Verification items for the finished model (mm, model axes). A direction names the side the tool comes from. Give positions to 0.01 mm unless a question says otherwise; leave off trailing zeros. Write each loop counter-clockwise with the first axis right and the second up, starting at its lowest first coordinate (ties: lowest second). Pieces come first, ordered by that corner, then holes. Notation, with made-up numbers: (13, 22.25) - (20, 22.25) arc R24 cw to (20, 56.25) - close; hole circle Ø10 at (-19.5, 53.5). An arc over 180 degrees is marked (long way). Put each result on its own line as item: value.
from build123d import *

# Parameters (mm, degrees)
IZIM1_R                     = 35
Y_KSEKLIK_EKSTR_ZYON1_DEPTH = 10
IZIM2_W                     = 12
IZIM2_H                     = 12
KES_EKSTR_ZYON1_DEPTH       = 16
RADYUS1_R                   = 3


with BuildPart() as part:
    # Çizim1 → Yükseklik-Ekstrüzyon1 (new body)
    with BuildSketch(Plane.XY):
        Circle(IZIM1_R)
    extrude(amount=Y_KSEKLIK_EKSTR_ZYON1_DEPTH)

    # Çizim2 → Kes-Ekstrüzyon1 (cut)
    with BuildSketch(Plane(origin=(0, 0, 0), x_dir=(-1, 0, 0), z_dir=(0, 0, -1))):
        with Locations((0, 29)):
            Rectangle(IZIM2_W, IZIM2_H)
        with Locations((0, -29)):
            Rectangle(IZIM2_W, IZIM2_H)
    extrude(amount=-KES_EKSTR_ZYON1_DEPTH, mode=Mode.SUBTRACT)

    # Radyus1
    radyus1_edges = [part.edges().sort_by_distance(p)[0] for p in [
        (-6, 34.481879299, 5),
        (6, 34.481879299, 5),
        (6, 23, 5),
        (-6, 23, 5),
        (-6, -34.481879299, 5),
        (-6, -23, 5),
        (6, -34.481879299, 5),
        (6, -23, 5),
    ]]
    fillet(radyus1_edges, radius=RADYUS1_R)


solid = part.part
Q1. Section check C-C, the plane x = -11.5. Record the cut outline in (y, z).
Answers follow:
outline: (-33.06, 0) - (33.06, 0) - (33.06, 10) - (-33.06, 10) - close
Q2. Go/stop test with flat-tipped pins: pin 1 Ø4 at (y, z) = (29, 3) entering from +X; pin 2 Ø5 at (y, z) = (27.5, 3.5) entering from -X; pin 3 Ø4 at (y, z) = (-27.5, 3.5) entering from +X. Record where each tip stops, or that it passes through.
Answers follow:
pin 1: stops at x = 22.27
pin 2: stops at x = -24.49
pin 3: stops at x = 23.97
Q3. Set-up check for faces 4 (the face through (-5.14, -23.9, 5.07)), 5 (the face through (0, 0, 10)), 6 (the face through (-6, 28, 5)): record each of +Z, -Z, +X, -X, +Y, -Y from which the full face is reachable in a straight line by a thin tool's end or side.
Answers follow:
face 4: +Z, -Z, -Y
face 5: +Z, +X, -X, +Y, -Y
face 6: +Z, -Z, +Y
Q4. Section check A-A, the plane z = 7. Record the cut outline in (x, y), plus the area to 3 significant figures.
Answers follow:
outline: (-9.84, -33.59) arc R3 ccw to (-6, -30.71) - (-6, -26) arc R3 cw to (-3, -23) - (3, -23) arc R3 cw to (6, -26) - (6, -30.71) arc R3 ccw to (9.84, -33.59) arc R35 ccw to (9.84, 33.59) arc R3 ccw to (6, 30.71) - (6, 26) arc R3 cw to (3, 23) - (-3, 23) arc R3 cw to (-6, 26) - (-6, 30.71) arc R3 ccw to (-9.84, 33.59) arc R35 ccw to start
area: 3,560 mm2
Q5. Scan lines: line 1 along X through (y, z) = (27, 4); line 2 along X through (y, z) = (-26, 9.75); line 3 along Y through (x, z) = (-26.5, 6.25). Record each from-to range of solid material in increasing order.
Answers follow:
line 1: x = -22.27 to -6, 6 to 22.27
line 2: x = -23.43 to -6, 6 to 23.43
line 3: y = -22.86 to 22.86
Q6. Section check B-B, the plane y = -7. Record the cut outline in (x, z), plus the area to 3 significant figures.
Answers follow:
outline: (-34.29, 0) - (34.29, 0) - (34.29, 10) - (-34.29, 10) - close
area: 686 mm2
Q7. Release check for a two-part mould opening along X. For faces 1 (the face through (5.1, -23.86, 5.07)), 2 (the face through (-34.994, 0.63, 4.93)), 3 (the face through (0, 0, 0)) record: released by +X, released by -X, zero draft, split by the parting line, or undercut.
Answers follow:
face 1: undercut
face 2: released by -X
face 3: zero draft
